Autodesk Inventor part; units mm, degrees
ref_plane "YZ Plane" through (0, 0, 0) normal (1, 0, 0) x (0, 1, 0)
ref_plane "XZ Plane" through (0, 0, 0) normal (0, 1, 0) x (-1, 0, 0)
ref_plane "XY Plane" through (0, 0, 0) normal (0, 0, 1) x (1, 0, 0)
sketch "Schizzo4" plane through (0, 0, 0) normal (0, 0, 1) x (1, 0, 0)
  line L0 (0, 0) -> (0, 68)
  line L1 (0, 68) -> (3.9, 68)
  line L2 (3.9, 68) -> (3.9, 5.2)
  line L3 (3.9, 5.2) -> (7.5, 5.2)
  line L4 (7.5, 5.2) -> (7.5, 0)
  line L5 (7.5, 0) -> (0, 0)
  dimension "d0" = 5.2
  dimension "d1" = 7.8
  dimension "d2" = 15
  dimension "d3" = 68
revolve "Rivoluzione1" add sketch "Schizzo4" angle 360 about axis through (0, 0, 0) along (0, 1, 0)
thread "Filettatura1"
sketch "Schizzo5" plane through (0, 0, 0) normal (0, -1, 0) x (1, 0, 0)
  line L0 (-3.6084, -6.25) -> (-7.2169, 0)
  line L1 (-7.2169, 0) -> (-3.6084, 6.25)
  line L2 (-3.6084, 6.25) -> (3.6084, 6.25)
  line L3 (3.6084, 6.25) -> (7.2169, 0)
  line L4 (7.2169, 0) -> (3.6084, -6.25)
  line L5 (3.6084, -6.25) -> (-3.6084, -6.25)
  circle A0 centre (0, 0) radius 7.5
  dimension "d9" = 12.5
extrude "Estrusione1" cut sketch "Schizzo5" against normal up to surface (5.2 mm away)
sketch "Schizzo6" plane through (0, 0, 0) normal (0, 0, 1) x (1, 0, 0)
  line L0 (3.9, 68) -> (-3.9, 68)
  line L1 (3.6, 68) -> (3.9, 67.7)
  line L2 (3.9, 5.2) -> (3.9, 68)
  line L3 (3.9, 68) -> (3.6, 68)
  line L4 (3.6084, 0) -> (7.2169, 0)
  line L5 (5.75, 0) -> (7.2169, 0.4)
  line L6 (7.2169, 0.4) -> (7.2169, 0)
  line L7 (7.2169, 0) -> (5.75, 0)
  line L8 (7.2169, 5.2) -> (3.6084, 5.2)
  line L9 (0, 0) -> (0, 68)
  dimension "d12" = 45
  dimension "d14" = 0.3
  dimension "d15" = 4.8
  dimension "d16" = 11.5
revolve "Rivoluzione3" cut sketch "Schizzo6" angle 360 about axis through (0, 0, 0) along (0, 1, 0)
properties part number "Bolt" material "Acciaio"
Here's how the part is built. I have some questions about the finished solid (model axes, mm). A direction names the side the tool comes from. Give positions to 0.01 mm unless a question says otherwise; leave off trailing zeros. Loops run counter-clockwise (first coordinate to the right, second up) from the corner with the lowest first, then second, coordinate; pieces in that order, holes last. Notation, with made-up numbers: M 27,3 L 61,3 A11 ccw 61,12 Z; hole C -19.5,18 d10. An arc over 180 degrees is marked long. Put each result on its own line as item: value. Start each with the question number.
(1) I need wall thicknesses on line 1 along Y through (x, z) = (4, 3.75); line 2 along Z through (x, y) = (1.5, 54); line 3 along Z through (x, y) = (6.25, 3.5). Which ranges of each line are inside material? Lowest first, please. Write a range as [from, to].
(2) I want a section at B-B on y = 20. Please give me the cut outline in (x, z).
(3) I want a section at A-A on x = 0. Please give me the cut outline in (y, z).
(4) For faces 4 (the flat face through (-5.387, 2.633, -3.169)), 5 (the flat face through (3, 5.2, -3)), which set-ups out of +Z, -Z, +X, -X, +Y, -Y let a thin tool reach every point of the face, with its end or its side?
(5) If we mould it in two halves opening along Y, with no side actions, what happens to faces 1 (the flat face through (0, 0, 0)), 2 (the flat face through (0, 68, 0)), 3 (the flat face through (-5.44, 2.63, 3.08))? For each: +Y half, -Y half, draft (parallel to the pull), parting line (faces both ways), or undercut.
(6) Will these pins go through, and if not, where does the flat tip stop? pin 1 Ø5 at (y, z) = (27.5, -2) entering from +X; pin 2 Ø3 at (x, y) = (4, 60.5) entering from -Z; pin 3 Ø6 at (x, y) = (4, 49) entering from +Z; pin 4 Ø2 at (y, z) = (17.5, 5) entering from -X.
Answer block:
1. line 1: [0, 5.2]
1. line 2: [-3.6, 3.6]
1. line 3: [-1.67, 1.67]
2. outline: C 0,0 d7.8
3. outline: M 0,-5.75 L 0.14,-6.25 L 5.2,-6.25 L 5.2,-3.9 L 67.7,-3.9 L 68,-3.6 L 68,3.6 L 67.7,3.9 L 5.2,3.9 L 5.2,6.25 L 0.14,6.25 L 0,5.75 Z
4. face 4: -Z, -X, +Y, -Y
4. face 5: +Y
5. face 1: -Y half
5. face 2: +Y half
5. face 3: draft
6. pin 1: x = 3.9
6. pin 2: z = -2.99
6. pin 3: z = 3.77
6. pin 4: through
